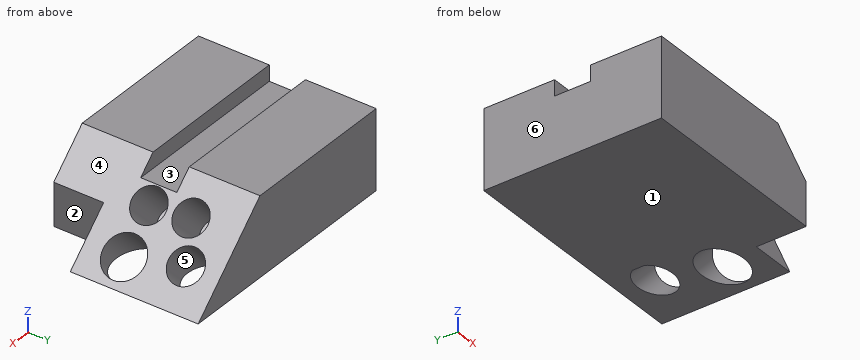
from build123d import *

# Parameters (mm, degrees)
F0_W      = 116.9611811638
F0_H      = 60.1601935923
F1_DEPTH  = 38.1
F3_DEPTH  = 31.75
F4_W      = 8.79971501
F4_H      = 17.4067560583
F4_W_2    = 75.7910068654
F5_DEPTH  = 7.62
F6_DEPTH  = 12.7
F7_DEPTH  = 12.7
F8_W      = 25.9574428201
F8_H      = 27.7897324413
F9_DEPTH  = 25.4
F10_R     = 8.1507716862
F11_DEPTH = 25.4
F12_R     = 8.1743450513
F13_DEPTH = 25.4
F14_R     = 10.0476315022
F15_DEPTH = 25.4
F16_R     = 8.34829694
F17_DEPTH = 25.4


with BuildPart() as f1:
    # F0 (on Top) → F1 (new body)
    with BuildSketch(Plane.XY):
        Rectangle(F0_W, F0_H)
    extrude(amount=F1_DEPTH)

    # F2 (on Front) → F3 (cut, symmetric)
    with BuildSketch(Plane.XZ):
        Polygon((13.2841020823, 43.822273612), (14.8110100999, 40.4630750418), (65.1989877224, -7.1764695458), (65.1989877224, 43.822273612), align=None)
    extrude(amount=F3_DEPTH, both=True, mode=Mode.SUBTRACT)

    # F4 (on face) → F5 (cut)
    with BuildSketch(Plane.XY.offset(38.1)):
        with Locations((21.7102737885, 0)):
            Rectangle(F4_W, F4_H)
        with Locations((-20.5850871492, 0)):
            Rectangle(F4_W_2, F4_H)
    extrude(amount=-F5_DEPTH, mode=Mode.SUBTRACT)

    # F6 (add): a face of the model
    f6_faces = [f1.faces().sort_by_distance(p)[0] for p in [
        (-9.8052950563, -30.0800967962, 17.7163922315),
    ]]
    extrude(f6_faces, amount=F6_DEPTH)

    # F7 (add): a face of the model
    f7_faces = [f1.faces().sort_by_distance(p)[0] for p in [
        (-9.8052950563, 30.0800967962, 17.7163922315),
    ]]
    extrude(f7_faces, amount=F7_DEPTH)

    # F8 (on Top) → F9 (cut)
    with BuildSketch(Plane.XY):
        with Locations((48.8610677421, -32.6758408919)):
            Rectangle(F8_W, F8_H)
    extrude(amount=F9_DEPTH, mode=Mode.SUBTRACT)

    # F10 (on face) → F11 (cut)
    with BuildSketch(Plane(origin=(27.1903243303, 0, 28.7589956151), x_dir=(0.7266466393, 0, -0.6870113985), z_dir=(0.6870113985, 0, 0.7266466393))):
        with Locations((4.6751173213, 19.3886086345)):
            Circle(F10_R)
    extrude(amount=-F11_DEPTH, mode=Mode.SUBTRACT)

    # F12 (on face) → F13 (cut)
    with BuildSketch(Plane(origin=(27.1903243303, 0, 28.7589956151), x_dir=(0.7266466393, 0, -0.6870113985), z_dir=(0.6870113985, 0, 0.7266466393))):
        with Locations((6.3146823086, 0)):
            Circle(F12_R)
    extrude(amount=-F13_DEPTH, mode=Mode.SUBTRACT)

    # F14 (on face) → F15 (cut)
    with BuildSketch(Plane(origin=(27.1903243303, 0, 28.7589956151), x_dir=(0.7266466393, 0, -0.6870113985), z_dir=(0.6870113985, 0, 0.7266466393))):
        with Locations((28.6077186465, 0)):
            Circle(F14_R)
    extrude(amount=-F15_DEPTH, mode=Mode.SUBTRACT)

    # F16 (on face) → F17 (cut)
    with BuildSketch(Plane(origin=(27.1903243303, 0, 28.7589956151), x_dir=(0.7266466393, 0, -0.6870113985), z_dir=(0.6870113985, 0, 0.7266466393))):
        with Locations((22.8316728026, 26.6705863178)):
            Circle(F16_R)
    extrude(amount=-F17_DEPTH, mode=Mode.SUBTRACT)


solid = f1.part
Work out the finished part from the listing and answer in its coordinate system (mm). Face numbers are marked on the shaded views. A direction names the side the tool comes from. Round coordinates to 2 decimals unless told otherwise and drop trailing zeros. Loops run counter-clockwise (first coordinate to the right, second up) from the corner with the lowest first, then second, coordinate; pieces in that order, holes last. Notation, with made-up numbers: (84.25, -29) - (129.25, -29) arc R20 cw to (129.25, -21) - close; hole circle Ø1 at (14, 71). An arc over 180 degrees is marked (long way). Use one line per item in the form item = value. Start each with the question number.
(1) Which of the six approach directions +Z, -Z, +X, -X, +Y, -Y give full straight-line access (tool end or side, diameter ignored) to the marked faces 1 and 2?
(2) Determine the mould class of the marked faces 3, 4, 5 and 6 for opening direction X: +X half, -X half, draft (parallel to the pull), parting line (faces both ways), or undercut.
(3) Find section A-A on y = 21. Determine the outline of the cut face in (x, z).
(4) Find section C-C on y = -23. Determine the outline of the cut face in (x, z), and give its area (3 significant figures).
(5) Flat-ended cylindrical pins translate along their axes: P1, Ø10.5, axis at x = 51, z = 12.5, coming from the -Y side; P2, Ø22.5, axis at y = -34.5, z = 12.5, coming from the +X side; P3, Ø12, axis at y = -28.5, z = 33.5, coming from the +X side. Find the tip coordinate at first contact, or state that the pin passes through.
(6) Consider line 1 (Y direction, x = -44.5, z = 36); line 2 (Y direction, x = 23.5, z = 15); line 3 (Z direction, x = -9, y = 1). Determine where each line is inside the solid, lowest interval first.
(7) Find section B-B on x = -15. Determine the outline of the cut face in (y, z).
(8) Find section D-D on z = 4. Give the number of separate pieces and of enclosed holes in the cut face, and give its area (3 significant figures).
Answer list:
q1.face_1 = -Z, +X, -X, +Y, -Y
q1.face_2 = +Z, -Z, +X, -Y
q2.face_3 = draft
q2.face_4 = +X half
q2.face_5 = undercut
q2.face_6 = -X half
q3.outline = (-58.48, 0) - (22.99, 0) - (39.33, 17.28) - (36.39, 20.06) - (18.94, 1.6) - (7.33, 12.58) - (24.78, 31.04) - (17.31, 38.1) - (-58.48, 38.1) - close; (39.85, 0) - (57.61, 0) - (48.23, 8.86) - close
q4.outline = (-58.48, 0) - (35.88, 0) - (35.88, 20.54) - (17.31, 38.1) - (-58.48, 38.1) - close
q4.area = 3,430 mm^2
q5.P1 = -18.78
q5.P2 = 35.88
q5.P3 = 28.52
q6.line_1 = -42.78 to -8.7, 8.7 to 42.78
q6.line_2 = -42.78 to -8.16, 8.16 to 11.51, 27.27 to 42.78
q6.line_3 = 0 to 30.48
q7.outline = (-42.78, 0) - (42.78, 0) - (42.78, 38.1) - (8.7, 38.1) - (8.7, 30.48) - (-8.7, 30.48) - (-8.7, 38.1) - (-42.78, 38.1) - close
q8.separate_pieces = 1
q8.enclosed_holes = 3
q8.area = 8,320 mm^2
